The listing builds one solid part. Answer for the finished solid, in the listing's coordinates (mm). Round coordinates to 2 decimals unless told otherwise and drop trailing zeros. Write each loop counter-clockwise with the first axis right and the second up, starting at its lowest first coordinate (ties: lowest second). Pieces come first, ordered by that corner, then holes. Notation, with made-up numbers: (14.5, 73.5) - (53.5, 73.5) arc R28 ccw to (53.5, 103.5) - close; hole circle Ø4 at (39, 73.25). An arc over 180 degrees is marked (long way). Answer in a Markdown table with one row per item.
from build123d import *

# Parameters (mm, degrees)
F0_R     = 11.049
F1_DEPTH = 6.35


with BuildPart() as f1:
    # F0 (on Top) → F1 (new body)
    with BuildSketch(Plane.XY):
        with BuildLine():
            ThreePointArc((0, 11.049), (-7.812823, -7.812823), (11.049, 0))
            ThreePointArc((11.049, 0), (7.812823, 7.812823), (0, 11.049))
        make_face()
        with BuildLine():
            ThreePointArc((11.049, 30.48), (-7.812823, 38.292823), (0, 19.431))
            ThreePointArc((0, 19.431), (7.812823, 22.667177), (11.049, 30.48))
        make_face()
        with BuildLine():
            ThreePointArc((20.388099, -27.851922), (39.467067, -20.17153), (30.216541, -1.802447))
            ThreePointArc((30.216541, -1.802447), (27.230144, 17.407217), (13.926422, 31.582573))
            ThreePointArc((13.926422, 31.582573), (-2.264476, 44.265247), (-13.547306, 27.069516))
            ThreePointArc((-13.547306, 27.069516), (-28.690164, 14.878388), (-34.314522, -3.730651))
            ThreePointArc((-34.314522, -3.730651), (-37.202591, -24.093718), (-16.669235, -25.267069))
            ThreePointArc((-16.669235, -25.267069), (1.46002, -32.285604), (20.388099, -27.851922))
        make_face()
        with Locations((-26.396454, -15.24)):
            Circle(F0_R, mode=Mode.SUBTRACT)
        with BuildLine():
            ThreePointArc((-24.710147, -1.37215), (-20.709724, 7.796596), (-10.767389, 8.9008))
            ThreePointArc((-10.767389, 8.9008), (-13.767563, -2.369623), (-7.172004, -11.988463))
            Line((-7.172004, -11.988463), (-12.78411, -12.099142))
            ThreePointArc((-12.78411, -12.099142), (-17.054117, -4.853392), (-24.710147, -1.37215))
        make_face(mode=Mode.SUBTRACT)
        with BuildLine():
            ThreePointArc((13.548183, -23.867834), (15.3921, -25.055532), (15.5478, -27.24332))
            ThreePointArc((15.5478, -27.24332), (0.143167, -29.572149), (-14.195671, -23.479213))
            Line((-14.195671, -23.479213), (-6.069518, -16.243227))
            ThreePointArc((-6.069518, -16.243227), (2.250939, -23.885085), (13.548183, -23.867834))
        make_face(mode=Mode.SUBTRACT)
        with Locations((26.396454, -15.24)):
            Circle(F0_R, mode=Mode.SUBTRACT)
        with BuildLine():
            Line((13.968316, -0.216906), (16.870219, -5.021793))
            ThreePointArc((16.870219, -5.021793), (12.730219, -12.342602), (13.54339, -20.71354))
            ThreePointArc((13.54339, -20.71354), (3.602811, -21.833445), (-2.324624, -13.775232))
            ThreePointArc((-2.324624, -13.775232), (8.935935, -10.738248), (13.968316, -0.216906))
        make_face(mode=Mode.SUBTRACT)
        with BuildLine():
            ThreePointArc((0, 11.049), (7.812823, 7.812823), (11.049, 0))
            ThreePointArc((11.049, 0), (-7.812823, -7.812823), (0, 11.049))
        make_face(mode=Mode.SUBTRACT)
        with BuildLine():
            ThreePointArc((-27.444242, 0.200847), (-29.394777, -0.802184), (-31.367307, 0.15687))
            ThreePointArc((-31.367307, 0.15687), (-25.681816, 14.662088), (-13.235759, 24.033418))
            Line((-13.235759, 24.033418), (-11.032288, 13.37797))
            ThreePointArc((-11.032288, 13.37797), (-21.81056, 9.993172), (-27.444242, 0.200847))
        make_face(mode=Mode.SUBTRACT)
        with BuildLine():
            ThreePointArc((13.092013, 4.874432), (7.97073, 11.47294), (0, 13.97))
            ThreePointArc((0, 13.97), (-3.510832, 13.521648), (-6.796312, 12.20537))
            Line((-6.796312, 12.20537), (-4.086109, 17.120935))
            ThreePointArc((-4.086109, 17.120935), (-2.065764, 16.663578), (0, 16.51))
            ThreePointArc((0, 16.51), (6.240688, 17.981412), (11.166757, 22.08569))
            ThreePointArc((11.166757, 22.08569), (17.106913, 14.036849), (13.092013, 4.874432))
        make_face(mode=Mode.SUBTRACT)
        with BuildLine():
            ThreePointArc((13.896059, 23.666987), (14.002677, 25.857716), (15.819507, 27.08645))
            ThreePointArc((15.819507, 27.08645), (25.538649, 14.910061), (27.43143, -0.554205))
            Line((27.43143, -0.554205), (17.101806, 2.865257))
            ThreePointArc((17.101806, 2.865257), (19.559621, 13.891913), (13.896059, 23.666987))
        make_face(mode=Mode.SUBTRACT)
        with BuildLine():
            ThreePointArc((11.049, 30.48), (7.812823, 22.667177), (0, 19.431))
            ThreePointArc((0, 19.431), (-7.812823, 38.292823), (11.049, 30.48))
        make_face(mode=Mode.SUBTRACT)
    extrude(amount=F1_DEPTH)


solid = f1.part
(1) Section D-D (x = 21.5) is taken. Give the vertices of the cut face in (y, z).
Checked values:
| item | result |
|---|---|
| outline | (-28.32, 0) - (-25.14, 0) - (-25.14, 6.35) - (-28.32, 6.35) - close; (-5.34, 0) - (1.41, 0) - (1.41, 6.35) - (-5.34, 6.35) - close; (21.7, 0) - (25.66, 0) - (25.66, 6.35) - (21.7, 6.35) - close |
(2) Section C-C (y = 35) is taken. Give the vertices of the cut face in (x, z).
Checked values:
| item | result |
|---|---|
| outline | (-13.22, 0) - (-10.08, 0) - (-10.08, 6.35) - (-13.22, 6.35) - close; (10.08, 0) - (13.22, 0) - (13.22, 6.35) - (10.08, 6.35) - close |
(3) Flat-ended cylindrical pins translate along their axes: pin 1 (1.5 mm diameter, centred on y = 18.5, z = 5, fed in from -X); pin 2 (6 mm diameter, centred on x = -18.5, y = -23, fed in from -Z); pin 3 (20 mm diameter, centred on x = -26.4, y = -15.24, fed in from -Z); pin 4 (3 mm diameter, centred on x = -22, z = 2, fed in from +Y). Find the tip coordinate at first contact, or state that the pin passes through.
Checked values:
| item | result |
|---|---|
| pin 1 | stops at x = -26.52 |
| pin 2 | stops at z = 0 |
| pin 3 | passes through |
| pin 4 | stops at y = 23.28 |
(4) Section B-B (y = -15.24) is taken. Give the vertices of the cut face in (x, z), and give its area (3 significant figures).
Checked values:
| item | result |
|---|---|
| outline | (-40.37, 0) - (-37.45, 0) - (-37.45, 6.35) - (-40.37, 6.35) - close; (-15.35, 0) - (-2.05, 0) - (-2.05, 6.35) - (-15.35, 6.35) - close; (12.43, 0) - (15.35, 0) - (15.35, 6.35) - (12.43, 6.35) - close; (37.45, 0) - (40.37, 0) - (40.37, 6.35) - (37.45, 6.35) - close |
| area | 140 mm2 |
(5) For a pull along Y with two mould halves and no side action, classify faces 1 (the cylindrical face through (1.184, -32.265, 3.131)), 2 (the cylindrical face through (25.452, 15.113, 3.131)) as pulls with the +Y half, pulls with the -Y half, needs draft (parallel to the pull), parting line crosses it, or undercut.
Checked values:
| item | result |
|---|---|
| face 1 | pulls with the -Y half |
| face 2 | undercut |
(6) Find the intervals of material crossed by line 1 (X direction, y = -23.5, z = 4.5); line 2 (Y direction, x = 0, z = 4.75); line 3 (Y direction, x = -17, z = 2) (3 decimals), in increasing order.
Checked values:
| item | result |
|---|---|
| line 1 | x = -37.66 to -33.73, -19.06 to -14.17, 1.35 to 19.06, 33.73 to 37.66 |
| line 2 | y = -32.15 to -29.55, -22.79 to -19.16, -13.97 to -11.05, 11.05 to 13.97, 16.51 to 19.43, 41.53 to 44.45 |
| line 3 | y = -25.578 to -21.053, -9.427 to -4.902, 9.495 to 12.616, 22.25 to 25.461 |
(7) Section A-A (x = 32) is taken. Give the vertices of the cut face in (y, z).
Checked values:
| item | result |
|---|---|
| outline | (-28.04, 0) - (-24.76, 0) - (-24.76, 6.35) - (-28.04, 6.35) - close; (-5.72, 0) - (-2.44, 0) - (-2.44, 6.35) - (-5.72, 6.35) - close |
